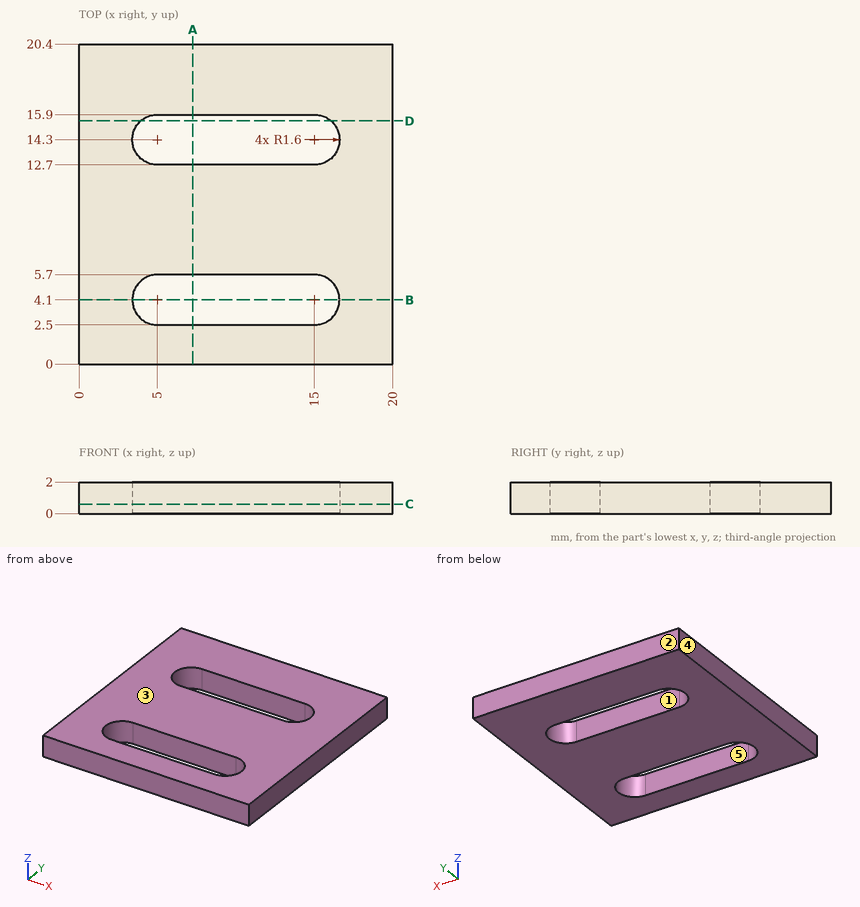
For this review, use the dimensioned drawing (mm, ordinates from the lowest corner) and the shaded views. A direction names the side the tool comes from. Round coordinates to 2 decimals unless told otherwise and drop trailing zeros. Write each loop counter-clockwise with the first axis right and the second up, starting at its lowest first coordinate (ties: lowest second). Pieces come first, ordered by that corner, then holes. Notation, with made-up numbers: M -7.75,68.25 L 9.25,68.25 A18 ccw 9.25,91.25 Z; hole C 56.25,-17 d11. An arc over 180 degrees is marked long. Write item = value, one per line. Start each with the question number.
(1) We need section D-D (y = 15.5). Give the boundary of the cut face in (x, z).
(2) For line 1 along Y through (x, z) = (10.5, 0.15); line 2 along X through (y, z) = (13, 1); line 3 along X through (y, z) = (14.75, 0.7), list the stretches that pass through material, from the lowest coordinate up.
(3) We need section B-B (y = 4.1). Give the boundary of the cut face in (x, z), then the cut area to 3 significant figures.
(4) For the marked faces 1 and 2, list the 3-axis set-ups (+Z, -Z, +X, -X, +Y, -Y) from which the entire face can be reached by the end or side of a thin tool; tool diameter is ignored.
(5) We need section C-C (z = 0.6). Give the boundary of the cut face in (x, y), then the cut area to 3 significant figures.
(6) We need section A-A (x = 7.25). Give the boundary of the cut face in (y, z), then the cut area to 3 significant figures.
(7) The part is to be moulded in two halves that separate along X. For the marked faces 3, 4 and 5, say which applies: +X half, -X half, draft (parallel to the pull), parting line (faces both ways), or undercut.
Results found:
q1.outline = M 0,0 L 3.94,0 L 3.94,2 L 0,2 Z; M 16.06,0 L 20,0 L 20,2 L 16.06,2 Z
q2.line_1 = 0 to 2.5, 5.7 to 12.7, 15.9 to 20.4
q2.line_2 = 0 to 4.07, 15.93 to 20
q2.line_3 = 0 to 3.46, 16.54 to 20
q3.outline = M 0,0 L 3.4,0 L 3.4,2 L 0,2 Z; M 16.6,0 L 20,0 L 20,2 L 16.6,2 Z
q3.area = 13.6 mm²
q4.face_1 = +Z, -Z
q4.face_2 = +Z, -Z, +X, -X, +Y
q5.outline = M 0,0 L 20,0 L 20,20.4 L 0,20.4 Z; hole M 5,2.5 L 15,2.5 A1.6 ccw 15,5.7 L 5,5.7 A1.6 ccw Z; hole M 5,12.7 L 15,12.7 A1.6 ccw 15,15.9 L 5,15.9 A1.6 ccw Z
q5.area = 328 mm²
q6.outline = M 0,0 L 2.5,0 L 2.5,2 L 0,2 Z; M 5.7,0 L 12.7,0 L 12.7,2 L 5.7,2 Z; M 15.9,0 L 20.4,0 L 20.4,2 L 15.9,2 Z
q6.area = 28.0 mm²
q7.face_3 = draft
q7.face_4 = -X half
q7.face_5 = undercut
